```python
from build123d import *

# Parameters (mm, degrees)
SKETCH1_W            = 95
SKETCH1_H            = 40
BOSS_EXTRUDE1_DEPTH  = 5
SKETCH2_W            = 14.5
SKETCH2_H            = 6
BOSS_EXTRUDE2_DEPTH  = 32
SKETCH4_R            = 2.75
CUT_EXTRUDE1_DEPTH   = 6
BOSS_EXTRUDE5_DEPTH  = 32
SKETCH11_W           = 4.5
SKETCH11_H           = 37
BOSS_EXTRUDE6_DEPTH  = 75
SKETCH12_R           = 4
CUT_EXTRUDE3_DEPTH   = 110
BOSS_EXTRUDE9_DEPTH  = 4
SKETCH16_R           = 11.3
SKETCH16_R_2         = 1
BOSS_EXTRUDE11_DEPTH = 8
SKETCH17_R           = 5.912080619
BOSS_EXTRUDE12_DEPTH = 50


with BuildPart() as part:
    # Sketch1 → Boss-Extrude1 (new body)
    with BuildSketch(Plane(origin=(0, 0, 0), x_dir=(1, 0, 0), z_dir=(0, 1, 0))):
        Rectangle(SKETCH1_W, SKETCH1_H)
    extrude(amount=BOSS_EXTRUDE1_DEPTH)

    # Sketch2 → Boss-Extrude2 (add)
    with BuildSketch(Plane(origin=(0, 5, 0), x_dir=(1, 0, 0), z_dir=(0, 1, 0))):
        with Locations((-40.25, 17)):
            Rectangle(SKETCH2_W, SKETCH2_H)
        with Locations((40.25, 17)):
            Rectangle(SKETCH2_W, SKETCH2_H)
    extrude(amount=BOSS_EXTRUDE2_DEPTH)

    # Sketch4 → Cut-Extrude1 (cut)
    with BuildSketch(Plane(origin=(0, 0, -20), x_dir=(-1, 0, 0), z_dir=(0, 0, -1))):
        with Locations((37.5, 11.5)):
            Circle(SKETCH4_R)
        with Locations((37.5, 28.5)):
            Circle(SKETCH4_R)
        with Locations(Location((-37.5, 28.5, 0), (0, 0, 180))):
            Circle(SKETCH4_R)
        with Locations(Location((-37.5, 11.5, 0), (0, 0, 180))):
            Circle(SKETCH4_R)
    extrude(amount=-CUT_EXTRUDE1_DEPTH, mode=Mode.SUBTRACT)

    # Sketch10 → Boss-Extrude5 (add)
    with BuildSketch(Plane(origin=(0, 5, 0), x_dir=(1, 0, 0), z_dir=(0, 1, 0))):
        Polygon((-47.5, -14), (-47.5, -20), (-43.5, -20), (43.5, -20), (47.5, -20), (47.5, -19), (47.5, 14), (43.5, 14), (43.5, -14), (-43.5, -14), (-43.5, 14), (-47.5, 14), align=None)
    extrude(amount=BOSS_EXTRUDE5_DEPTH)

    # Sketch11 → Boss-Extrude6 (add)
    with BuildSketch(Plane.XY.offset(20)):
        with Locations((-45.25, 18.5)):
            Rectangle(SKETCH11_W, SKETCH11_H)
        with Locations((45.25, 18.5)):
            Rectangle(SKETCH11_W, SKETCH11_H)
    extrude(amount=BOSS_EXTRUDE6_DEPTH)

    # Sketch12 → Cut-Extrude3 (cut)
    with BuildSketch(Plane.ZY.offset(47.5)):
        with Locations((77, 18.5)):
            Circle(SKETCH12_R)
    extrude(amount=-CUT_EXTRUDE3_DEPTH, mode=Mode.SUBTRACT)

    # Sketch15 → Boss-Extrude9 (add)
    with BuildSketch(Plane(origin=(0, 37, 0), x_dir=(1, 0, 0), z_dir=(0, 1, 0))):
        Polygon((28.857864376, -20), (43, -34.142135624), (43, -20), align=None)
        Polygon((-28.857864376, -20), (-43, -20), (-43, -34.142135624), align=None)
    boss_extrude9 = extrude(amount=-BOSS_EXTRUDE9_DEPTH)

    # Mirror2: Boss-Extrude9 across plane
    add(boss_extrude9.mirror(Plane.ZX.offset(18.5)))

    # Sketch16 → Boss-Extrude11 (add)
    with BuildSketch(Plane(origin=(47.5, 0, 0), x_dir=(0, 0, -1), z_dir=(1, 0, 0))):
        with BuildLine():
            Line((-66.888373029, 4.145732342), (-69.234713241, 6.492072554))
            ThreePointArc((-69.234713241, 6.492072554), (-77, 4.2), (-84.765286759, 6.492072554))
            Line((-84.765286759, 6.492072554), (-87.111626971, 4.145732342))
            ThreePointArc((-87.111626971, 4.145732342), (-91.354267658, 4.145732342), (-91.354267658, 8.388373029))
            Line((-91.354267658, 8.388373029), (-89.007927446, 10.734713241))
            ThreePointArc((-89.007927446, 10.734713241), (-91.3, 18.5), (-89.007927446, 26.265286759))
            Line((-89.007927446, 26.265286759), (-91.354267658, 28.611626971))
            ThreePointArc((-91.354267658, 28.611626971), (-91.354267658, 32.854267658), (-87.111626971, 32.854267658))
            Line((-87.111626971, 32.854267658), (-84.765286759, 30.507927446))
            ThreePointArc((-84.765286759, 30.507927446), (-77, 32.8), (-69.234713241, 30.507927446))
            Line((-69.234713241, 30.507927446), (-66.888373029, 32.854267658))
            ThreePointArc((-66.888373029, 32.854267658), (-62.645732342, 32.854267658), (-62.645732342, 28.611626971))
            Line((-62.645732342, 28.611626971), (-64.992072554, 26.265286759))
            ThreePointArc((-64.992072554, 26.265286759), (-62.7, 18.5), (-64.992072554, 10.734713241))
            Line((-64.992072554, 10.734713241), (-62.645732342, 8.388373029))
            ThreePointArc((-62.645732342, 8.388373029), (-62.645732342, 4.145732342), (-66.888373029, 4.145732342))
        make_face()
        with Locations((-77, 18.5)):
            Circle(SKETCH16_R, mode=Mode.SUBTRACT)
        with Locations((-64.767052685, 6.267052685)):
            Circle(SKETCH16_R_2, mode=Mode.SUBTRACT)
        with Locations((-89.232947315, 6.267052685)):
            Circle(SKETCH16_R_2, mode=Mode.SUBTRACT)
        with Locations((-89.232947315, 30.732947315)):
            Circle(SKETCH16_R_2, mode=Mode.SUBTRACT)
        with Locations((-64.767052685, 30.732947315)):
            Circle(SKETCH16_R_2, mode=Mode.SUBTRACT)
    extrude(amount=BOSS_EXTRUDE11_DEPTH)

    # Sketch17 → Boss-Extrude12 (add)
    with BuildSketch(Plane(origin=(0, 0, 14), x_dir=(-1, 0, 0), z_dir=(0, 0, -1))):
        with Locations((0, 19)):
            Circle(SKETCH17_R)
    extrude(amount=BOSS_EXTRUDE12_DEPTH)


solid = part.part
```
Source: CAD feature listing. Evaluate the final solid. Frame: model axes, mm. A direction names the side the tool comes from. Give positions to 0.01 mm unless a question says otherwise; leave off trailing zeros. Loops run counter-clockwise (first coordinate to the right, second up) from the corner with the lowest first, then second, coordinate; pieces in that order, holes last. Notation, with made-up numbers: M -31,49.5 L -8,49.5 A12 ccw -8,63.5 Z; hole C 62,15 d9. An arc over 180 degrees is marked long. Put each result on its own line as item: value.
Q1. Line query: probe 1 along Y at (x, z) = (44, 77); probe 2 along X at (y, z) = (4.5, 22); probe 3 along X at (y, z) = (5.5, 62). Output: solid intervals per line, ascending. Write a range as [from, to].
Response values:
probe 1: y = [0, 14.5], [22.5, 37]
probe 2: x = [-47.5, -43], [43, 47.5]
probe 3: x = [-47.5, -43], [43, 55.5]
Q2. Section D-D (z = 37). Return the cut outline in (x, y), and give its area (3 significant figures).
Response values:
outline: M -47.5,0 L -43,0 L -43,37 L -47.5,37 Z; M 43,0 L 47.5,0 L 47.5,37 L 43,37 Z
area: 333 mm²
Q3. Pin query (flat end, axial travel): P1, Ø1.5, axis at x = 21.5, y = 14.5, coming from the -Z side; P2, Ø18.5, axis at x = 20.5, y = 24.5, coming from the +Z side; P3, Ø3, axis at y = 29, z = -18.5, coming from the +X side. Return the tip coordinate at first contact, or that it passes through.
Response values:
P1: stops at z = 14
P2: stops at z = 20
P3: stops at x = 47.5
Q4. Section B-B (z = 77). Return the cut outline in (x, y), and give its area (3 significant figures).
Response values:
outline: M -47.5,0 L -43,0 L -43,14.5 L -47.5,14.5 Z; M -47.5,22.5 L -43,22.5 L -43,37 L -47.5,37 Z; M 43,0 L 47.5,0 L 47.5,4.2 L 55.5,4.2 L 55.5,7.2 L 47.5,7.2 L 47.5,14.5 L 43,14.5 Z; M 43,22.5 L 47.5,22.5 L 47.5,29.8 L 55.5,29.8 L 55.5,32.8 L 47.5,32.8 L 47.5,37 L 43,37 Z
area: 309 mm²
Q5. Reachability of faces 4 (the flat face through (33, 21, -17)), 5 (the cylindrical face through (34.753, 11.379, -17.042)), 6 (the flat face through (39, 4, 24)), 7 (the cylindrical face through (51.44, 21.89, 66.22)), 8 (the cylindrical face through (51.4, 4.2, 76.9)) from +Z, -Z, +X, -X, +Y, -Y: full face, straight path, thin tool, end or side. Return the list, or none.
Response values:
face 4: -Z, +Y
face 5: -Z
face 6: +Z
face 7: +X
face 8: +X, -Y
Q6. Mould query, pull axis Y, two halves, no side actions, for faces 1 (the cylindrical face through (51.4, 18.6, 62.7)), 2 (the flat face through (35.83, 35.03, 26.97)), 3 (the flat face through (0, 37, 16)). Classes: released by +Y, released by -Y, zero draft, split by the parting line, or undercut.
Response values:
face 1: undercut
face 2: zero draft
face 3: released by +Y
Q7. Section C-C (x = 0). Return the cut outline in (y, z).
Response values:
outline: M 0,-20 L 5,-20 L 5,14 L 13.09,14 L 13.09,-36 L 24.91,-36 L 24.91,14 L 37,14 L 37,20 L 0,20 Z
Q8. Section A-A (z = -17). Return the cut outline in (x, y).
Response values:
outline: M -47.5,0 L 47.5,0 L 47.5,37 L 33,37 L 33,5 L -33,5 L -33,37 L -47.5,37 Z; C 0,19 d11.82; hole C -37.5,11.5 d5.5; hole C -37.5,28.5 d5.5; hole C 37.5,11.5 d5.5; hole C 37.5,28.5 d5.5
